Input: part model. Units: mm. Frame: model coordinates. Face numbers are marked on the shaded views. A direction names the side the tool comes from. Give positions to 0.01 mm unless a question says otherwise; leave off trailing zeros. Loops run counter-clockwise (first coordinate to the right, second up) from the corner with the lowest first, then second, coordinate; pieces in that order, holes last. Notation, with made-up numbers: M 28.25,-15.75 L 53.25,-15.75 A19 cw 53.25,-6.75 Z; hole C 27,23.5 d7. An arc over 180 degrees is marked long. Use a Markdown table: item, result. Add a question column.
from build123d import *

# Parameters (mm, degrees)
SZKIC2_W                    = 5.611911117
SZKIC2_H                    = 18
WYTNIJ_WYCI_GNI_CIE3_DEPTH  = 200
SZKIC3_R                    = 4
WYTNIJ_WYCI_GNI_CIE4_DEPTH  = 9
WYTNIJ_WYCI_GNI_CIE5_DEPTH  = 1
SZKIC5_R                    = 2.025
DODANIE_WYCI_GNI_CIE1_DEPTH = 25


with BuildPart() as part:
    # Szkic1 → Obrót1 (revolve)
    with BuildSketch(Plane.XY):
        with BuildLine():
            Line((0, 0), (-2, 0))
            Line((-2, 0), (-2, 1.009242946))
            Line((-2, 1.009242946), (-3.014835025, 1.009242946))
            Line((-3.014835025, 1.009242946), (-3.014835025, 1.600524218))
            Line((-3.014835025, 1.600524218), (-2, 1.600524218))
            Line((-2, 1.600524218), (-2, 45))
            Line((-2, 45), (-4, 45))
            Line((-4, 45), (-4, 50))
            Line((-4, 50), (-3, 50))
            Line((-3, 50), (-3, 73.52))
            Line((-3, 73.52), (-6.811196546, 80.121186056))
            ThreePointArc((-6.811196546, 80.121186056), (-8.18368509, 89.74931215), (0, 95.004008644))
            Line((0, 95.004008644), (0, 88.504008644))
            ThreePointArc((0, 88.504008644), (-2.5, 86.004008644), (0, 83.504008644))
            Line((0, 83.504008644), (0, 0))
        make_face()
    revolve(axis=Axis((0, 83.504008644, 0), (0, -1, 0)))

    # Szkic2 → Wytnij-wyciągnięcie3 (cut)
    with BuildSketch(Plane(origin=(0, 0, 0), x_dir=(1, 0, 0), z_dir=(0, 1, 0))):
        with Locations((-6.805955559, 0)):
            Rectangle(SZKIC2_W, SZKIC2_H)
        with Locations((6.805955559, 0)):
            Rectangle(SZKIC2_W, SZKIC2_H)
    extrude(amount=WYTNIJ_WYCI_GNI_CIE3_DEPTH, mode=Mode.SUBTRACT)

    # Szkic3 → Wytnij-wyciągnięcie4 (cut, through all)
    with BuildSketch(Plane.ZY.offset(4)):
        with Locations((0, 86.004008644)):
            Circle(SZKIC3_R)
    extrude(amount=-WYTNIJ_WYCI_GNI_CIE4_DEPTH, mode=Mode.SUBTRACT)

    # Szkic4 → Wytnij-wyciągnięcie5 (cut)
    with BuildSketch(Plane.ZY.offset(4)):
        with BuildLine():
            ThreePointArc((6.270693727, 79.461614917), (-1.54e-07, 95.066266393), (-6.270693505, 79.461614705))
            add(Edge.make_bspline(
                [(-6.270693505, 79.461614705), (-5.860155238, 78.888013675), (-5.439822901, 78.322282195), (-4.56334323, 77.21959664), (-4.106381954, 76.681557874), (-3.363374021, 75.926338216), (-3.10680463, 75.684743321), (-2.565651322, 75.233486624), (-2.278481074, 75.02263049), (-1.674076312, 74.662473364), (-1.356546022, 74.513041633), (-0.676664628, 74.303793525), (-0.328815369, 74.249380941), (0.202925796, 74.253535488), (0.380729476, 74.269527018), (0.727839454, 74.32754423), (0.898553898, 74.369864163), (1.234860958, 74.478505876), (1.400715996, 74.545180561), (1.719331355, 74.695600019), (1.873358854, 74.779672361), (2.32266111, 75.053340603), (2.606912587, 75.265451803), (3.145505929, 75.720013642), (3.399015103, 75.960994151), (4.130320647, 76.709293024), (4.580547786, 77.240534568), (5.447234702, 78.332319258), (5.863652605, 78.892898741), (6.270693727, 79.461614917)],
                knots=[0, 0, 0, 0, 0.125, 0.125, 0.25, 0.25, 0.3125, 0.3125, 0.375, 0.375, 0.4375, 0.4375, 0.5, 0.5, 0.53125, 0.53125, 0.5625, 0.5625, 0.59375, 0.59375, 0.625, 0.625, 0.6875, 0.6875, 0.75, 0.75, 0.875, 0.875, 1, 1, 1, 1], degree=3))
        make_face()
    wytnij_wyci_gni_cie5 = extrude(amount=-WYTNIJ_WYCI_GNI_CIE5_DEPTH, mode=Mode.SUBTRACT)

    # Lustro1: Wytnij-wyciągnięcie5 across plane
    add(wytnij_wyci_gni_cie5.mirror(Plane(origin=(0, 0, 0), x_dir=(0, 0, 1), z_dir=(1, 0, 0))), mode=Mode.SUBTRACT)

    # Szkic5 → Dodanie-wyciągnięcie1 (add)
    with BuildSketch(Plane.XZ.offset(-45)):
        Circle(SZKIC5_R)
    extrude(amount=DODANIE_WYCI_GNI_CIE1_DEPTH)


solid = part.part
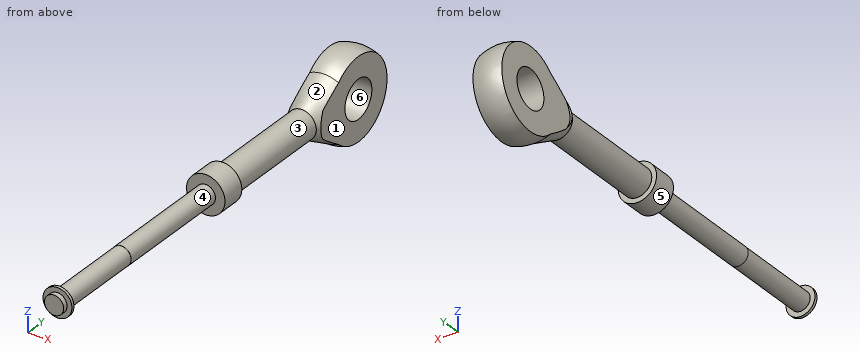
1) Section query C-C, the plane y = 25.5. Return the cut outline in (x, z) (3 decimals), and give its area (3 significant figures).
2) Ray query, line 1 (Y direction, x = 0.5, z = -0.25); line 2 (Y direction, x = -2.5, z = 1.25); line 3 (Z direction, x = 0.25, y = 61.5). Return the intervals inside material, ascending. Write a range as [from, to].
3) Pull-direction query (Y, two-part tool) for the marked faces 1, 2 and 3; classes: pulls with the +Y half, pulls with the -Y half, needs draft (parallel to the pull), parting line crosses it, or undercut.
4) Section query A-A, the plane x = 0. Return the cut outline in (y, z) (3 decimals).
5) Reachability of the marked faces 4, 5 and 6 from +Z, -Z, +X, -X, +Y, -Y: full face, straight path, thin tool, end or side. Return the list, or none.
6) Contact query for flat-ended pins moving along their axis: P1, Ø3, axis at x = 2, y = 41, coming from the -Z side; P2, Ø3, axis at y = 42, z = 4.5, coming from the -X side; P3, Ø2, axis at x = -2.5, z = 0, coming from the +Y side; P4, Ø9, axis at y = 86, z = 0, coming from the -X side. Output: stop coordinate, or through.
7) Section query B-B, the plane y = 65. Return the cut outline in (x, z), and give its area (3 significant figures).
Entries:
| question | item | result |
|---|---|---|
| 1 | outline | C 0,0 d4.05 |
| 1 | area | 12.9 mm² |
| 2 | line 1 | y = [0, 82.01], [90, 94.99] |
| 2 | line 2 | y = [1.01, 1.6], [45, 82.2], [89.8, 94.56] |
| 2 | line 3 | z = [-2.99, 2.99] |
| 3 | face 1 | needs draft |
| 3 | face 2 | undercut |
| 3 | face 3 | undercut |
| 4 | outline | M 0,-2 L 1.009,-2 L 1.009,-3.015 L 1.601,-3.015 L 1.601,-2 L 20,-2 L 20,-2.025 L 45,-2.025 L 45,-4 L 50,-4 L 50,-3 L 73.52,-3 L 80.121,-6.811 A9 ccw long 80.121,6.811 L 73.52,3 L 50,3 L 50,4 L 45,4 L 45,2.025 L 20,2.025 L 20,2 L 1.601,2 L 1.601,3.015 L 1.009,3.015 L 1.009,2 L 0,2 Z; hole C 86.004,0 d8 |
| 5 | face 4 | none |
| 5 | face 5 | -Y |
| 5 | face 6 | +X, -X |
| 6 | P1 | stops at z = -1.96 |
| 6 | P2 | passes through |
| 6 | P3 | stops at y = 94.88 |
| 6 | P4 | stops at x = -3 |
| 7 | outline | C 0,0 d6 |
| 7 | area | 28.3 mm² |
